Read the model definition and answer for the solid it produces. Units are mm, in the model's axes. Face numbers are marked on the shaded views. A direction names the side the tool comes from. Coordinates: 2 decimals unless noted, no trailing zeros. Loops run counter-clockwise (first coordinate to the right, second up) from the corner with the lowest first, then second, coordinate; pieces in that order, holes last. Notation, with made-up numbers: (35.5, -30) - (43.5, -30) arc R17 ccw to (43.5, -10) - close; hole circle Ø1 at (85.5, -13.5). An arc over 180 degrees is marked (long way). Use one line per item in the form item = value.
Autodesk Inventor part; units mm, degrees
ref_plane "Work Plane1" through (0, 0, 3) normal (0, 0, -1) x (-1, 0, 0)
ref_plane "YZ Plane" through (0, 0, 0) normal (1, 0, 0) x (0, 1, 0)
ref_plane "XZ Plane" through (0, 0, 0) normal (0, 1, 0) x (-1, 0, 0)
sketch "Sketch1" plane through (0, 0, 0) normal (0, 0, 1) x (1, 0, 0)
  line L0 (0, 0) -> (10, 0)
  line L1 (10, 0) -> (10, 10)
  line L2 (10, 10) -> (0, 10)
  line L3 (0, 10) -> (0, 0)
  dimension "d0" = 10
  dimension "d1" = 10
extrude "Extrusion1" add sketch "Sketch1" along normal blind 9
sketch "Sketch2" plane through (10, 0, 0) normal (1, 0, 0) x (0, 0, -1)
  circle A0 centre (-15, 5) radius 5 construction
  line L0 (0, 0) -> (0, 10)
  arc A1 (-15, 10) -> (-15, 0) centre (-15, 5) ccw
  line L1 (-9, 0) -> (-9, 10)
  line L2 (-15, 10) -> (-9, 10)
  line L3 (-15, 0) -> (-9, 0)
  circle A2 centre (-15, 5) radius 1.5
  point P0 (0, 5)
  dimension "d4" = 10
  dimension "d5" = 15
  dimension "d6" = 3
extrude "Extrusion2" add sketch "Sketch2" against normal blind 3
sketch "Sketch3" plane through (0, 0, 0) normal (-1, 0, 0) x (0, 0, 1)
  circle A0 centre (15, 5) radius 1.5
  arc A1 (15, 0) -> (15, 10) centre (15, 5) ccw
  line L0 (15, 10) -> (9, 10)
  line L1 (9, 0) -> (9, 10)
  line L2 (9, 0) -> (15, 0)
  point P0 (0, 0)
extrude "Extrusion3" add sketch "Sketch3" against normal blind 3
fillet "Fillet1" radius 2 6 edges at (0, 5, 20) (0, 0, 7.5) (0, 10, 7.5) (10, 5, 20) (10, 0, 7.5) (10, 10, 7.5)
sketch "Sketch4" plane through (0, 0, 0) normal (0, 0, -1) x (-1, 0, 0)
  circle A0 centre (-5, 5) radius 2
  line L0 (-8, 10) -> (-2, 10)
  line L1 (0, 8) -> (0, 2)
  point P0 (0, 0)
  point P1 (-5, 10)
  point P2 (0, 5)
  dimension "d12" = 4
extrude "Extrusion4" cut sketch "Sketch4" against normal through all
ref_plane "Work Plane1" through (0, 0, 3) normal (0, 0, -1) x (-1, 0, 0)
sketch "Sketch5" plane through (0, 0, 3) normal (0, 0, -1) x (-1, 0, 0)
  circle A0 centre (-5, 5) radius 2
  circle A1 centre (-5, 5) radius 3
  point P0 (0, 0)
  dimension "d16" = 6
extrude "Extrusion5" cut sketch "Sketch5" against normal through all
sketch "Sketch8" plane through (0, 2, 0) normal (-1, 0, 0) x (0, 0, 1)
  circle A0 centre (15, 3) radius 1.5
  circle A1 centre (15, 3) radius 3
  point P0 (0, -2)
  dimension "d20" = 6
extrude "Extrusion6" cut sketch "Sketch8" against normal blind 1
properties part number "Arm3" material "ABS Plastic"
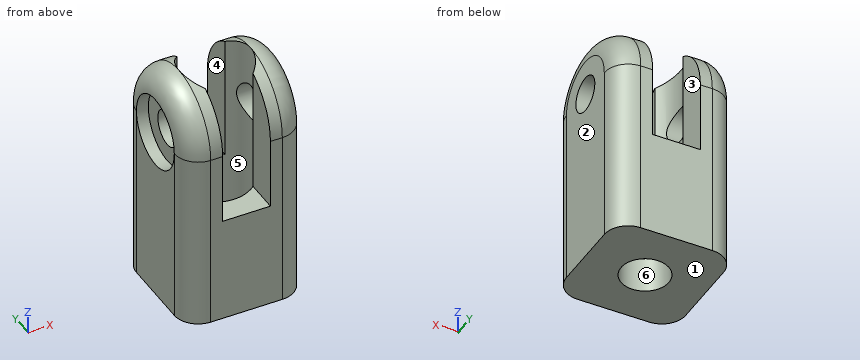
Item 1: The part is cut by section A-A on x = 5. Give the vertices of the cut face in (y, z).
Results below:
outline = (0, 0) - (3, 0) - (3, 3) - (2, 3) - (2, 9) - (0, 9) - close; (7, 0) - (10, 0) - (10, 9) - (8, 9) - (8, 3) - (7, 3) - close
Item 2: Find the intervals of material crossed by L1, parallel to Y at x = 2.05, z = 15; L2, parallel to X at y = 5, z = 8.5; L3, parallel to X at y = 5.25, z = 16.75, in increasing order.
Results below:
L1 = 0 to 3.5, 6.5 to 10
L2 = 0 to 2, 8 to 10
L3 = 1 to 2.01, 7.99 to 10
Item 3: The part is cut by section C-C on z = 3.5. Give the vertices of the cut face in (x, y).
Results below:
outline = (0, 2) arc R2 ccw to (2, 0) - (8, 0) arc R2 ccw to (10, 2) - (10, 8) arc R2 ccw to (8, 10) - (2, 10) arc R2 ccw to (0, 8) - close; hole circle Ø6 at (5, 5)
Item 4: For a pull along X with two mould halves and no side action, classify the marked faces 1, 2 and 3 as +X half, -X half, draft (parallel to the pull), parting line (faces both ways), or undercut.
Results below:
face_1 = draft
face_2 = +X half
face_3 = undercut
Item 5: Which of the six approach directions +Z, -Z, +X, -X, +Y, -Y give full straight-line access (tool end or side, diameter ignored) to the marked faces 4, 5 and 6?
Results below:
face_4 = +Z, +Y, -Y
face_5 = +Z
face_6 = +Z, -Z
Item 6: The part is cut by section B-B on z = 11.75. Give the vertices of the cut face in (x, y), plus the area to 3 significant figures.
Results below:
outline = (0, 2) arc R2 ccw to (2, 0) - (3, 0) - (3, 2.76) arc R3 cw to (3, 7.24) - (3, 10) - (2, 10) arc R2 ccw to (0, 8) - close; (7, 0) - (8, 0) arc R2 ccw to (10, 2) - (10, 8) arc R2 ccw to (8, 10) - (7, 10) - (7, 7.24) arc R3 cw to (7, 2.76) - close
area = 50.4 mm²
Item 7: The part is cut by section D-D on y = 4. Count the separate pieces of the cut face and the enclosed holes in it, plus the area to 3 significant figures.
Results below:
separate_pieces = 4
enclosed_holes = 0
area = 78.1 mm²
Item 8: Each of these flat-tipped pins is pushed along its axis until it touches: P1, Ø4, axis at x = 3.5, y = 1.5, coming from the +Z side; P2, Ø1.4, axis at y = 9, z = 16, coming from the +X side; P3, Ø3, axis at y = 6, z = 16, coming from the -X side. Where does it stop, or does it pass through?
Results below:
P1 = 19.69
P2 = 9.95
P3 = 1
